```python
from build123d import *

# Parameters (mm, degrees)
LINEAR_AUSTRAGEN_D_NN1_DEPTH                = 100
AUFSATZ_LINEAR_AUSTRAGEN3_REACH             = 160.325
AUFSATZ_LINEAR_START                        = 29
SKIZZE6_W                                   = 25
SKIZZE6_H                                   = 15
FASE1_SIZE                                  = 18
SKIZZE7_R                                   = 2.65
SCHNITT_LINEAR_AUSTRAGEN3_DEPTH             = 130.325171564
SCHNITT_LINEAR_START                        = -5
SCHNITT_LINEAR_AUSTRAGEN5_DEPTH             = 90
VERRUNDUNG1_R                               = 5
AUFSATZ_LINEAR_AUSTRAGEN5_REACH             = 131.325
AUFSATZ_LINEAR_AUSTRAGEN5_DIRECTION_2_REACH = 131.325


with BuildPart() as part:
    # Skizze1 → Linear-Austragen-Dünn1 (new body)
    with BuildSketch(Plane.XY):
        with BuildLine():
            Line((-33.2, -65), (0, -65))
            Line((0, -65), (33.2, -65))
            ThreePointArc((33.2, -65), (35.179898987, -64.179898987), (36, -62.2))
            Line((36, -62.2), (36, -38.522720569))
            ThreePointArc((36, -38.522720569), (36.601418547, -35.107070313), (38.333333333, -32.10226714))
            ThreePointArc((38.333333333, -32.10226714), (49.970076451, -1.729583607), (40.461208274, 29.375))
            ThreePointArc((40.461208274, 29.375), (36.91044215, 32.409264841), (32.368966619, 33.5))
            Line((32.368966619, 33.5), (0, 33.5))
            Line((0, 33.5), (-32.368966619, 33.5))
            ThreePointArc((-32.368966619, 33.5), (-36.91044215, 32.409264841), (-40.461208274, 29.375))
            ThreePointArc((-40.461208274, 29.375), (-49.970076451, -1.729583607), (-38.333333333, -32.10226714))
            ThreePointArc((-38.333333333, -32.10226714), (-36.601418547, -35.107070313), (-36, -38.522720569))
            Line((-36, -38.522720569), (-36, -62.2))
            ThreePointArc((-36, -62.2), (-35.179898987, -64.179898987), (-33.2, -65))
        make_face()
        with BuildLine():
            Line((-33.2, -62.51), (0, -62.51))
            Line((0, -62.51), (33.2, -62.51))
            ThreePointArc((33.2, -62.51), (33.419203102, -62.419203102), (33.51, -62.2))
            Line((33.51, -62.2), (33.51, -38.522720569))
            ThreePointArc((33.51, -38.522720569), (34.261171765, -34.2565734), (36.424333333, -30.503574237))
            ThreePointArc((36.424333333, -30.503574237), (47.481566644, -1.643450344), (38.446240102, 27.912125))
            ThreePointArc((38.446240102, 27.912125), (35.779614743, 30.190857895), (32.368966619, 31.01))
            Line((32.368966619, 31.01), (0, 31.01))
            Line((0, 31.01), (-32.368966619, 31.01))
            ThreePointArc((-32.368966619, 31.01), (-35.779614743, 30.190857895), (-38.446240102, 27.912125))
            ThreePointArc((-38.446240102, 27.912125), (-47.481566644, -1.643450344), (-36.424333333, -30.503574237))
            ThreePointArc((-36.424333333, -30.503574237), (-34.261171765, -34.2565734), (-33.51, -38.522720569))
            Line((-33.51, -38.522720569), (-33.51, -62.2))
            ThreePointArc((-33.51, -62.2), (-33.419203102, -62.419203102), (-33.2, -62.51))
        make_face(mode=Mode.SUBTRACT)
    extrude(amount=LINEAR_AUSTRAGEN_D_NN1_DEPTH)

    # Austragung2: sweep along a path in Skizze16
    with BuildLine(Plane.XY.offset(100)) as austragung2_path:
        Line((33.51, -62.2), (33.51, -38.522720569))
        ThreePointArc((33.51, -38.522720569), (34.261171765, -34.2565734), (36.424333333, -30.503574237))
        ThreePointArc((36.424333333, -30.503574237), (47.481566644, -1.643450344), (38.446240102, 27.912125))
        ThreePointArc((38.446240102, 27.912125), (35.779614743, 30.190857895), (32.368966619, 31.01))
        Line((32.368966619, 31.01), (-32.368966619, 31.01))
        ThreePointArc((-32.368966619, 31.01), (-35.779614743, 30.190857895), (-38.446240102, 27.912125))
        ThreePointArc((-38.446240102, 27.912125), (-47.481566644, -1.643450344), (-36.424333333, -30.503574237))
        ThreePointArc((-36.424333333, -30.503574237), (-34.261171765, -34.2565734), (-33.51, -38.522720569))
        Line((-33.51, -38.522720569), (-33.51, -62.2))
    # Skizze17 → Austragung2 (sweep)
    with BuildSketch(Plane(origin=(0, 0, 0), x_dir=(0, 0, -1), z_dir=(1, 0, 0))):
        Polygon((-100, 31.01), (-100, 29.01), (-98, 29.01), (-96, 31.01), align=None)
    sweep(path=austragung2_path.line)

    # Skizze6 → Aufsatz-Linear austragen3 (add, up to next)
    with BuildSketch(Plane(origin=(0, 0, 0), x_dir=(0, 0, -1), z_dir=(1, 0, 0)).offset(AUFSATZ_LINEAR_START), mode=Mode.PRIVATE) as aufsatz_linear_austragen3_sk1:
        with Locations((-87.5, 0)):
            Rectangle(SKIZZE6_W, SKIZZE6_H)
    aufsatz_linear_austragen3_tool1 = extrude(aufsatz_linear_austragen3_sk1.sketch, amount=AUFSATZ_LINEAR_AUSTRAGEN3_REACH, mode=Mode.PRIVATE) - part.part
    # Skizze6 → Aufsatz-Linear austragen3 (add, up to next)
    with BuildSketch(Plane(origin=(0, 0, 0), x_dir=(0, 0, -1), z_dir=(1, 0, 0)).offset(AUFSATZ_LINEAR_START), mode=Mode.PRIVATE) as aufsatz_linear_austragen3_sk2:
        with Locations((-12.5, 0)):
            Rectangle(SKIZZE6_W, SKIZZE6_H)
    aufsatz_linear_austragen3_tool2 = extrude(aufsatz_linear_austragen3_sk2.sketch, amount=AUFSATZ_LINEAR_AUSTRAGEN3_REACH, mode=Mode.PRIVATE) - part.part
    aufsatz_linear_austragen3_1 = aufsatz_linear_austragen3_tool1.solids().sort_by_distance((29, 0, 87.5))[0]
    add(aufsatz_linear_austragen3_1)
    aufsatz_linear_austragen3_2 = aufsatz_linear_austragen3_tool2.solids().sort_by_distance((29, 0, 12.5))[0]
    add(aufsatz_linear_austragen3_2)
    aufsatz_linear_austragen3 = aufsatz_linear_austragen3_1 + aufsatz_linear_austragen3_2  # Aufsatz-Linear austragen3 as one shape, for the pattern or mirror that repeats it

    # Spiegeln1: Aufsatz-Linear austragen3 across plane
    add(aufsatz_linear_austragen3.mirror(Plane(origin=(0, 0, 0), x_dir=(0, 0, 1), z_dir=(1, 0, 0))))

    # Fase1
    fase1_edges = [part.edges().sort_by_distance(p)[0] for p in [
        (29, 0, 75),
        (-29, 0, 75),
        (29, 0, 25),
        (-29, 0, 25),
    ]]
    chamfer(fase1_edges, length=FASE1_SIZE)

    # Skizze7 → Schnitt-Linear austragen3 (cut, through all)
    with BuildSketch(Plane.XY.offset(100)):
        with Locations((-35, 0)):
            Circle(SKIZZE7_R)
        with Locations((35, 0)):
            Circle(SKIZZE7_R)
    extrude(amount=-SCHNITT_LINEAR_AUSTRAGEN3_DEPTH, mode=Mode.SUBTRACT)

    # Skizze9 → Schnitt-Linear austragen5 (cut)
    with BuildSketch(Plane.XY.offset(100).offset(SCHNITT_LINEAR_START)):
        Polygon((-39.618802154, 0), (-37.309401077, -4), (-32.690598923, -4), (-30.381197846, 0), (-32.690598923, 4), (-37.309401077, 4), align=None)
        Polygon((30.381197846, 0), (32.690598923, -4), (37.309401077, -4), (39.618802154, 0), (37.309401077, 4), (32.690598923, 4), align=None)
    extrude(amount=-SCHNITT_LINEAR_AUSTRAGEN5_DEPTH, mode=Mode.SUBTRACT)

    # Verrundung1
    verrundung1_edges = [part.edges().sort_by_distance(p)[0] for p in [
        (-46.914284605, 7.5, 85.542857697),
        (-29, 7.5, 96.5),
        (-29, -7.5, 96.5),
        (-46.914284605, -7.5, 85.542857697),
        (46.914284605, -7.5, 85.542857697),
        (29, -7.5, 96.5),
        (29, 7.5, 96.5),
        (46.914284605, 7.5, 85.542857697),
        (-46.914284605, -7.5, 12.457142303),
        (-29, -7.5, 3.5),
        (-29, 7.5, 3.5),
        (-46.914284605, 7.5, 12.457142303),
        (46.914284605, -7.5, 12.457142303),
        (29, -7.5, 3.5),
        (29, 7.5, 3.5),
        (46.914284605, 7.5, 12.457142303),
    ]]
    fillet(verrundung1_edges, radius=VERRUNDUNG1_R)

    # Skizze17<3> → Aufsatz-Linear austragen5 (add, up to next)
    with BuildSketch(Plane(origin=(0, 0, 0), x_dir=(0, 0, -1), z_dir=(1, 0, 0)), mode=Mode.PRIVATE) as aufsatz_linear_austragen5_sk1:
        Polygon((-98, -60.51), (-96, -62.51), (-100, -62.51), (-100, -60.51), align=None)
    aufsatz_linear_austragen5_tool1 = extrude(aufsatz_linear_austragen5_sk1.sketch, amount=-AUFSATZ_LINEAR_AUSTRAGEN5_REACH, mode=Mode.PRIVATE) - part.part
    add(aufsatz_linear_austragen5_tool1.solids().sort_by_distance((0, -61.621111, 98.444444))[0])

    # Skizze17<3> → Aufsatz-Linear austragen5 direction 2 (add, up to next)
    with BuildSketch(Plane(origin=(0, 0, 0), x_dir=(0, 0, -1), z_dir=(1, 0, 0)), mode=Mode.PRIVATE) as aufsatz_linear_austragen5_direction_2_sk1:
        Polygon((-98, -60.51), (-96, -62.51), (-100, -62.51), (-100, -60.51), align=None)
    aufsatz_linear_austragen5_direction_2_tool1 = extrude(aufsatz_linear_austragen5_direction_2_sk1.sketch, amount=AUFSATZ_LINEAR_AUSTRAGEN5_DIRECTION_2_REACH, mode=Mode.PRIVATE) - part.part
    add(aufsatz_linear_austragen5_direction_2_tool1.solids().sort_by_distance((0, -61.621111, 98.444444))[0])


solid = part.part
```
Build history of the part. All positions in model axes, mm. A direction names the side the tool comes from. Coordinates: 2 decimals unless noted, no trailing zeros. Order: outer loops, then holes, each group sorted by start corner. A loop starts at its lowest first (then second) coordinate and runs counter-clockwise, first axis right, second up.
Item 1: Mould opens along Z. For faces 1 (the flat face through (-40, 0, 18)), 2 (the flat face through (33.51, -51, 47)) say: released by +Z, released by -Z, zero draft, split by the parting line, or undercut.
Filled in:
face 1: undercut
face 2: zero draft
Item 2: Tool access for faces 3 (the cylindrical face through (44.69, -9.58, 11.77)), 4 (the flat face through (-31.52, 1.97, 92.83)), 5 (the flat face through (36, -51, 49)), 6 (the flat face through (37, 7.5, 7)): list every direction of +Z, -Z, +X, -X, +Y, -Y with a clear straight run to the whole face (end or side of a thin tool).
Filled in:
face 3: -Z
face 4: none
face 5: +Z, -Z, +X, -Y
face 6: +Z, -Z
Item 3: Drill centre lines: L1, parallel to Y at x = 32.5, z = 31; L2, parallel to X at y = -57.5, z = 39.5; L3, parallel to Y at x = -35, z = 98.75. Where is each one in solid material? Low to high.
Filled in:
L1: y = -65 to -62.51, 31.01 to 33.5
L2: x = -36 to -33.51, 33.51 to 36
L3: y = -64.34 to -29.09, -7.5 to -2.65, 2.65 to 7.5, 28.34 to 33.15
Item 4: Drop flat-ended pins along their axis: pin 1 Ø5 at (y, z) = (15.5, 62.5) entering from -X; pin 2 Ø5 at (y, z) = (5, 51.5) entering from +X; pin 3 Ø6 at (y, z) = (-37.5, 69.5) entering from +X. Give the stop position or say it passes through.
Filled in:
pin 1: stops at x = -48.28
pin 2: stops at x = 49.94
pin 3: stops at x = 36.84
Item 5: Saw through at A-A on x = 9. List the corners of the cut face in (y, z), then the cut area to 3 significant figures.
Filled in:
outline: (-65, 0) - (-62.51, 0) - (-62.51, 96) - (-60.51, 98) - (-60.51, 100) - (-65, 100) - close; (29.01, 98) - (31.01, 96) - (31.01, 0) - (33.5, 0) - (33.5, 100) - (29.01, 100) - close
area: 510 mm2
Item 6: Saw through at B-B on y = -59. List the corners of the cut face in (x, z), then the cut area to 3 significant figures.
Filled in:
outline: (-36, 0) - (-33.51, 0) - (-33.51, 96) - (-31.51, 98) - (-31.51, 100) - (-36, 100) - close; (31.51, 98) - (33.51, 96) - (33.51, 0) - (36, 0) - (36, 100) - (31.51, 100) - close
area: 510 mm2
Item 7: Saw through at C-C on z = 70. List the corners of the cut face in (x, y) (3 decimals).
Filled in:
outline: (-40.461, 29.375) arc R50 ccw to (-38.333, -32.102) arc R10 cw to (-36, -38.523) - (-36, -62.2) arc R2.8 ccw to (-33.2, -65) - (33.2, -65) arc R2.8 ccw to (36, -62.2) - (36, -38.523) arc R10 cw to (38.333, -32.102) arc R50 ccw to (40.461, 29.375) arc R10 ccw to (32.369, 33.5) - (-32.369, 33.5) arc R10 ccw to start; hole (-38.446, 27.912) arc R47.51 ccw to (-36.424, -30.504) arc R12.49 cw to (-33.51, -38.523) - (-33.51, -62.2) arc R0.31 ccw to (-33.2, -62.51) - (33.2, -62.51) arc R0.31 ccw to (33.51, -62.2) - (33.51, -38.523) arc R12.49 cw to (36.424, -30.504) arc R47.51 ccw to (38.446, 27.912) arc R7.51 ccw to (32.369, 31.01) - (-32.369, 31.01) arc R7.51 ccw to start
Item 8: Saw through at D-D on y = 5.5. List the corners of the cut face in (x, z).
Filled in:
outline: (-49.7, 0) - (-30, 0) - (-30, 8) - (-47, 25) - (-47.19, 25) - (-47.19, 75) - (-47, 75) - (-30, 92) - (-30, 100) - (-49.7, 100) - close; (30, 0) - (49.7, 0) - (49.7, 100) - (30, 100) - (30, 92) - (47, 75) - (47.19, 75) - (47.19, 25) - (47, 25) - (30, 8) - close
